The model under review builds one solid part; all positions refer to its coordinate system, in mm. A direction names the side the tool comes from. Coordinates: 2 decimals unless noted, no trailing zeros. Order: outer loops, then holes, each group sorted by start corner. A loop starts at its lowest first (then second) coordinate and runs counter-clockwise, first axis right, second up. Notation, with made-up numbers: (71, 34.25) -> (107, 34.25) arc R23 ccw to (107, 50.25) -> close; hole circle Ø10 at (16, 56.25). An arc over 180 degrees is marked (long way). Use one line per item in the form item = value. Start each with the question number.
(1) For faces 1 (the cylindrical face through (17.405, -0.867, -3.905)), 2 (the flat face through (-3, 0, -6.5)), list the 3-axis set-ups (+Z, -Z, +X, -X, +Y, -Y) from which the entire face can be reached by the end or side of a thin tool; tool diameter is ignored.
(2) Wall thickness on line 1 along X through (y, z) = (-0.75, -5.5); line 2 along Z through (x, y) = (19, -0.25): over which ranges is each line inside the solid? List them lowest first.
(3) Take a section at A-A (x = 3.5). State the section outline as (y, z) points.
(4) Insertion check: pin 1 Ø4 at (x, y) = (18.5, 5.5) entering from +Z; pin 2 Ø1.5 at (x, z) = (22, -5) entering from -Y; pin 3 Ø4 at (x, z) = (27.5, 4.5) entering from -Y; pin 4 Ø6 at (x, y) = (28, 1) entering from +Z. Each pin has a flat end and moves straight along its axis. Give the tip position at first contact, or say it passes through.
Autodesk Inventor part; units mm, degrees
ref_plane "Work Plane1" through (1.525, 0, 0) normal (0, 0, 1) x (1, 0, 0)
ref_plane "YZ Plane" through (0, 0, 0) normal (1, 0, 0) x (0, 1, 0)
ref_plane "XZ Plane" through (0, 0, 0) normal (0, 1, 0) x (-1, 0, 0)
sketch "Sketch1" plane through (0, 0, 0) normal (0, 0, 1) x (1, 0, 0)
  line L0 (0, 4) -> (35, 4)
  line L1 (35, 4) -> (35, 0)
  line L2 (35, 0) -> (0, 0)
  line L3 (-7, 0) -> (42, 0)
  line L4 (0, -0.8) -> (0, 4.8)
  line L5 (0, 4) -> (0, 0)
  dimension "d2" = 8
  dimension "d59" = 35
revolve "Body" add sketch "Sketch1" angle 360 about axis through (35, 0, 0) along (-1, 0, 0)
sketch "Sketch2" plane through (0, 0, 0) normal (-1, 0, 0) x (0, 0, 1)
  line L0 (0, 7.5056) -> (6.5, 3.7528)
  line L1 (6.5, 3.7528) -> (6.5, -3.7528)
  line L2 (6.5, -3.7528) -> (0, -7.5056)
  line L3 (0, -7.5056) -> (-6.5, -3.7528)
  line L4 (-6.5, -3.7528) -> (-6.5, 3.7528)
  line L5 (-6.5, 3.7528) -> (0, 7.5056)
  line L6 (-9.1, 0) -> (9.1, 0)
  line L7 (0, 10.5078) -> (0, -10.5078)
  point P0 (0, 0)
  point P1 (0, 0)
  dimension "d11" = 13
extrude "Head" add sketch "Sketch2" along normal blind 5.68
sketch "Sketch4" plane through (0, 0, 0) normal (0, 0, 1) x (1, 0, 0)
  line L0 (-4.9294, 7.8) -> (-5.68, 6.5)
  line L1 (-1.1, 0) -> (-0.234, 0)
  line L2 (-6.7692, 0) -> (0.8552, 0)
  line L3 (-5.68, 7.8) -> (-4.9294, 7.8)
  line L4 (-5.68, 6.5) -> (-5.68, 7.8)
  line L5 (0, 9.36) -> (0, -1.56)
  dimension "d65" = 13
  dimension "d67" = 30
  dimension "d68" = 15.6
  dimension "d69" = 5.68
revolve "Chamfer1" cut sketch "Sketch4" angle 360 about axis through (-1.1, 0, 0) along (1, 0, 0)
thread "Thread"
chamfer "Chamfer2" distance 0.7668 distance2 0.7669 1 edges at (35, -4, 0) measured on face at (35, -0.3588, 0.308)
fillet "Fillet" radius 0.1 1 edges at (0, -4, 0)
ref_plane "Work Plane1" through (1.525, 0, 0) normal (0, 0, 1) x (1, 0, 0)
equation "\"d2\" = GD"
equation "\"d59\" = NLG"
equation "\"d11\" = SW"
equation "\"d3\" = KOH"
equation "\"d15\" = GEL"
equation "\"d6\" = -0.5 * SPD + 0.5 * GD"
equation "\"d71\" = RR"
equation "\"d65\" = SW"
equation "\"d67\" = ANG1"
equation "\"d68\" = 1.2 * SW"
equation "\"d69\" = KOH"
equation "\"NLG\" = 35"
equation "\"GD\" = NND"
equation "\"BDM\" = NND"
equation "\"KOH\" = 5.68"
equation "\"GEL\" = 22"
equation "\"SW\" = 13"
equation "\"SW0\" = SW"
equation "\"SPD\" = NND - 1.2269 * PTC"
equation "\"SD2\" = NND"
equation "\"SD\" = 0"
equation "\"ANG1\" = 30deg"
equation "\"GAL\" = 0.61345 * PTC"
equation "\"GUL\" = 0.61345 * PTC"
equation "\"RR\" = 0.1"
equation "\"RR1\" = 0.4"
equation "\"GD1\" = THREADDIA - 1.2269 * PTC"
equation "\"THREADDIA\" = 8"
equation "\"TOA\" = 30deg"
equation "\"PTC\" = 1.25"
equation "\"KOH1\" = 3.7"
equation "\"NND\" = 8"
equation "\"E0\" = 1.155 * SW"
properties part number "ANSI B18.2.3.5M - M8 x 1.25 x 35" material "Steel, Mild"
Findings:
q1.face_1 = +X
q1.face_2 = -Z, +X, -X, +Y, -Y
q2.line_1 = -5.68 to 0
q2.line_2 = -3.99 to 3.99
q3.outline = circle Ø8 at (0, 0)
q4.pin_1 = 1.94
q4.pin_2 = through
q4.pin_3 = -3.12
q4.pin_4 = 4
